```python
from build123d import *

# Parameters (mm, degrees)
SKETCH1_R                   = 25.4
BOSS_EXTRUDE1_DEPTH         = 63.5
SKETCH2_R                   = 25.4
SKETCH2_R_2                 = 12.7
CUT_EXTRUDE1_DEPTH          = 114.3
SKETCH3_R                   = 4.7625
BOSS_EXTRUDE2_DEPTH         = 12.7
SKETCH4_R                   = 19.05
CUT_EXTRUDE2_DEPTH          = 2.54
F_3_8_16_TAPPED_HOLE1_D     = 7.9375
F_3_8_16_TAPPED_HOLE1_DEPTH = 26.924
F_3_8_16_TAPPED_HOLE1_TIP   = 2.384665582


with BuildPart() as part:
    # Sketch1 → Boss-Extrude1 (new body, symmetric)
    with BuildSketch(Plane(origin=(0, 0, 0), x_dir=(1, 0, 0), z_dir=(0, 1, 0))):
        Circle(SKETCH1_R)
    extrude(amount=BOSS_EXTRUDE1_DEPTH, both=True)

    # Sketch2 → Cut-Extrude1 (cut)
    with BuildSketch(Plane(origin=(0, 63.5, 0), x_dir=(1, 0, 0), z_dir=(0, 1, 0))):
        Circle(SKETCH2_R)
        Circle(SKETCH2_R_2, mode=Mode.SUBTRACT)
    extrude(amount=-CUT_EXTRUDE1_DEPTH, mode=Mode.SUBTRACT)

    # Sketch3 → Boss-Extrude2 (add)
    with BuildSketch(Plane(origin=(0, 63.5, 0), x_dir=(1, 0, 0), z_dir=(0, 1, 0))):
        Circle(SKETCH3_R)
    extrude(amount=BOSS_EXTRUDE2_DEPTH)

    # Sketch4 → Cut-Extrude2 (cut)
    with BuildSketch(Plane.XZ.offset(63.5)):
        Circle(SKETCH4_R)
    extrude(amount=-CUT_EXTRUDE2_DEPTH, mode=Mode.SUBTRACT)

    # 3/8-16 Tapped Hole1
    with Locations(Plane(origin=(0, -60.96, 0), x_dir=(-1, 0, 0), z_dir=(0, -1, 0))):
        with Locations((0, 0)):
            Hole(F_3_8_16_TAPPED_HOLE1_D / 2, depth=F_3_8_16_TAPPED_HOLE1_DEPTH)
            with Locations((0, 0, -(F_3_8_16_TAPPED_HOLE1_DEPTH + F_3_8_16_TAPPED_HOLE1_TIP / 2))):  # 118° drill point
                Cone(0, F_3_8_16_TAPPED_HOLE1_D / 2, F_3_8_16_TAPPED_HOLE1_TIP, mode=Mode.SUBTRACT)


solid = part.part
```
CAD build for the part. Positions are in the model's coordinates, mm. A direction names the side the tool comes from. Round coordinates to 2 decimals unless told otherwise and drop trailing zeros. Loops run counter-clockwise (first coordinate to the right, second up) from the corner with the lowest first, then second, coordinate; pieces in that order, holes last. Notation, with made-up numbers: M 70.25,-32 L 88.25,-32 A24 cw 88.25,-18 Z; hole C 44.25,-19.75 d9. An arc over 180 degrees is marked long. Return JSON: item names as keys, results as strings. Group by question number.
(1) Drop flat-ended pins along their axis: P1, Ø1, axis at y = -25.5, z = -14.5, coming from the -X side; P2, Ø5, axis at y = 43.5, z = 8.5, coming from the -X side; P3, Ø12, axis at x = 14, y = -15.5, coming from the -Z side; P4, Ø6, axis at x = 7, z = -7.5, coming from the -Y side. Give the stop position or say it passes through.
(2) Tool access for faces 1 (the flat face through (5, 63.5, 0)), 2 (the cylindrical face through (-0.86, -47.31, 3.874)), 3 (the flat face through (0, 76.2, 0)): list every direction of +Z, -Z, +X, -X, +Y, -Y with a clear straight run to the whole face (end or side of a thin tool).
(3) Saw through at B-B, the plane y = -36. List the corners of the cut face in (x, z), and give its area (3 significant figures).
(4) Saw through at A-A, the plane z = -9. List the corners of the cut face in (x, y).
(5) Saw through at D-D, the plane y = 44. List the corners of the cut face in (x, z), and give its area (3 significant figures).
(6) Mould opens along X. For faces 4 (the cylindrical face through (-3.78, 69.76, 2.9)), 5 (the flat face through (0, -60.96, 5)), 6 (the conical face through (0.51, -32.07, -0.47)), 7 (the flat face through (5, -50.8, -12)) say: +X half, -X half, draft (parallel to the pull), parting line (faces both ways), or undercut.
(7) Saw through at C-C, the plane x = -6.5. List the corners of the cut face in (y, z), and give its area (3 significant figures).
(8) Wall check: probe 1 along Z at (x, y) = (0, -40); probe 2 along Z at (x, y) = (0, -52); probe 3 along Y at (x, z) = (15.5, -18). Give the ranges that are in metal, low to high. Write a range as [from, to].
Answer list:
{
 "1": {"P1": "through", "P2": "x = -11.19", "P3": "z = -9.86", "P4": "y = -60.96"},
 "2": {"face 1": "+Y", "face 2": "-Y", "face 3": "+Z, -Z, +X, -X, +Y"},
 "3": {"outline": "C 0,0 d25.4; hole C 0,0 d7.94", "area": "457 mm2"},
 "4": {"outline": "M -23.75,-63.5 L -16.79,-63.5 L -16.79,-60.96 L 16.79,-60.96 L 16.79,-63.5 L 23.75,-63.5 L 23.75,-50.8 L 8.96,-50.8 L 8.96,63.5 L -8.96,63.5 L -8.96,-50.8 L -23.75,-50.8 Z"},
 "5": {"outline": "C 0,0 d25.4", "area": "507 mm2"},
 "6": {"face 4": "parting line", "face 5": "undercut", "face 6": "undercut", "face 7": "draft"},
 "7": {"outline": "M -63.5,-24.55 L -50.8,-24.55 L -50.8,-10.91 L 63.5,-10.91 L 63.5,10.91 L -50.8,10.91 L -50.8,24.55 L -63.5,24.55 L -63.5,17.91 L -60.96,17.91 L -60.96,-17.91 L -63.5,-17.91 Z", "area": "3,030 mm2"},
 "8": {"probe 1": "[-12.7, -3.97], [3.97, 12.7]", "probe 2": "[-25.4, -3.97], [3.97, 25.4]", "probe 3": "[-63.5, -50.8]"}
}
